```python
from build123d import *

# Parameters (mm, degrees)
F1_DEPTH = 1.5
F2_DEPTH = 0.5
F2_TAPER = 50
F3_DEPTH = 1.5


with BuildPart() as f1:
    # F0 (on Front) → F1 (new body)
    with BuildSketch(Plane.XZ):
        Polygon((-1.5, 1.5), (-20, 1.5), (-22.3259367049, 3), (-28.5, 0), (-22.3259367049, -3), (-20, -1.5), (-1.5, -1.5), (-1.5, -37), (-3, -39.3259400742), (0, -45.5), (3, -39.3259400742), (1.5, -37), (1.5, -1.5), (20, -1.5), (22.3259367049, -3), (28.5, 0), (22.3259367049, 3), (20, 1.5), (1.5, 1.5), (1.5, 23), (3, 25.3259400742), (0, 31.5), (-3, 25.3259400742), (-1.5, 23), align=None)
        Polygon((-1, -1), (-1.5, -1), (-20, -1), (-22.3259367049, -2.5), (-27.4709894508, 0), (-22.3259367049, 2.5), (-20, 1), (-1.5, 1), (-1, 1), (-1, 23), (-2.5, 25.3259400742), (0, 30.4709900124), (2.5, 25.3259400742), (1, 23), (1, 1), (1.5, 1), (20, 1), (22.3259367049, 2.5), (27.4709894508, 0), (22.3259367049, -2.5), (20, -1), (1.5, -1), (1, -1), (1, -37), (2.5, -39.3259400742), (0, -44.4709900124), (-2.5, -39.3259400742), (-1, -37), (-1, -1.5), align=None, mode=Mode.SUBTRACT)
        Polygon((-20, -1), (-1.5, -1), (-1, -1), (-1, -1.5), (-1, -37), (-2.5, -39.3259400742), (0, -44.4709900124), (2.5, -39.3259400742), (1, -37), (1, -1), (1.5, -1), (20, -1), (22.3259367049, -2.5), (27.4709894508, 0), (22.3259367049, 2.5), (20, 1), (1.5, 1), (1, 1), (1, 23), (2.5, 25.3259400742), (0, 30.4709900124), (-2.5, 25.3259400742), (-1, 23), (-1, 1), (-1.5, 1), (-20, 1), (-22.3259367049, 2.5), (-27.4709894508, 0), (-22.3259367049, -2.5), align=None)
    extrude(amount=F1_DEPTH)

    # F0 (on Front) → F2 (join)
    with BuildSketch(Plane.XZ):
        Polygon((-1.5, 1.5), (-20, 1.5), (-22.3259367049, 3), (-28.5, 0), (-22.3259367049, -3), (-20, -1.5), (-1.5, -1.5), (-1.5, -37), (-3, -39.3259400742), (0, -45.5), (3, -39.3259400742), (1.5, -37), (1.5, -1.5), (20, -1.5), (22.3259367049, -3), (28.5, 0), (22.3259367049, 3), (20, 1.5), (1.5, 1.5), (1.5, 23), (3, 25.3259400742), (0, 31.5), (-3, 25.3259400742), (-1.5, 23), align=None)
        Polygon((-1, -1), (-1.5, -1), (-20, -1), (-22.3259367049, -2.5), (-27.4709894508, 0), (-22.3259367049, 2.5), (-20, 1), (-1.5, 1), (-1, 1), (-1, 23), (-2.5, 25.3259400742), (0, 30.4709900124), (2.5, 25.3259400742), (1, 23), (1, 1), (1.5, 1), (20, 1), (22.3259367049, 2.5), (27.4709894508, 0), (22.3259367049, -2.5), (20, -1), (1.5, -1), (1, -1), (1, -37), (2.5, -39.3259400742), (0, -44.4709900124), (-2.5, -39.3259400742), (-1, -37), (-1, -1.5), align=None, mode=Mode.SUBTRACT)
        Polygon((-20, -1), (-1.5, -1), (-1, -1), (-1, -1.5), (-1, -37), (-2.5, -39.3259400742), (0, -44.4709900124), (2.5, -39.3259400742), (1, -37), (1, -1), (1.5, -1), (20, -1), (22.3259367049, -2.5), (27.4709894508, 0), (22.3259367049, 2.5), (20, 1), (1.5, 1), (1, 1), (1, 23), (2.5, 25.3259400742), (0, 30.4709900124), (-2.5, 25.3259400742), (-1, 23), (-1, 1), (-1.5, 1), (-20, 1), (-22.3259367049, 2.5), (-27.4709894508, 0), (-22.3259367049, -2.5), align=None)
    extrude(amount=-F2_DEPTH, taper=F2_TAPER)

    # F3 (add): a face of the model
    f3_faces = [f1.faces().sort_by_distance(p)[0] for p in [
        (0, -1.5, -4.093430874),
    ]]
    extrude(f3_faces, amount=F3_DEPTH)


solid = f1.part
```
Read the model definition and answer for the solid it produces. Units are mm, in the model's axes. A direction names the side the tool comes from. Coordinates: 2 decimals unless noted, no trailing zeros. Write each loop counter-clockwise with the first axis right and the second up, starting at its lowest first coordinate (ties: lowest second). Pieces come first, ordered by that corner, then holes. Notation, with made-up numbers: (-16.75, 21) - (-9.75, 21) arc R30 cw to (-9.75, 53) - close; hole circle Ø1 at (60.25, 20.25). An arc over 180 degrees is marked (long way). Answer as a JSON object with one key per item and string values. Group by question number.
1. Which of the six approach directions +Z, -Z, +X, -X, +Y, -Y give full straight-line access (tool end or side, diameter ignored) to faces 1 (the flat face through (-2.26, -1.48, 24.18)), 2 (the flat face through (2.24, -1.48, 24.15)), 3 (the flat face through (25.456, -1.479, 1.479)), 4 (the flat face through (21.18, -1.48, 2.26))?
2. Consider L1, parallel to X at y = -2.45, z = 2; L2, parallel to X at y = -1.75, z = -36. Determine where each line is inside the solid, lowest interval first. Write a range as [from, to].
3. A cutting plane is placed at A-A (y = -0.75). Determine the outline of the cut face in (x, z).
4. The mould has two halves that part along Z. Classify faces 5 (the flat face through (1.5, -1, -19)), 6 (the flat face through (-1.479, -1.479, 28.456)), 7 (the flat face through (0, -3, -4)), 8 (the flat face through (-25.456, -1.479, -1.479)): +Z half, -Z half, draft (parallel to the pull), parting line (faces both ways), or undercut.
5. Each of these flat-tipped pins is pushed along its axis until it touches: P1, Ø1.5, axis at x = 8.5, y = -2, coming from the -Z side; P2, Ø0.9, axis at y = -2, z = 16, coming from the +X side; P3, Ø1.5, axis at y = -2, z = 9.5, coming from the -X side. Where does it stop, or does it pass through?
Worked out:
{
 "1": {"face 1": "-X, +Y, -Y", "face 2": "+X, +Y, -Y", "face 3": "+Z, +X, +Y, -Y", "face 4": "+Z, +Y, -Y"},
 "2": {"L1": "x = [-24.38, -20.78], [-1.5, 1.5], [20.78, 24.38]", "L2": "x = [-1.5, 1.5]"},
 "3": {"outline": "(-28.5, 0) - (-22.33, -3) - (-20, -1.5) - (-1.5, -1.5) - (-1.5, -37) - (-3, -39.33) - (0, -45.5) - (3, -39.33) - (1.5, -37) - (1.5, -1.5) - (20, -1.5) - (22.33, -3) - (28.5, 0) - (22.33, 3) - (20, 1.5) - (1.5, 1.5) - (1.5, 23) - (3, 25.33) - (0, 31.5) - (-3, 25.33) - (-1.5, 23) - (-1.5, 1.5) - (-20, 1.5) - (-22.33, 3) - close"},
 "4": {"face 5": "undercut", "face 6": "+Z half", "face 7": "draft", "face 8": "-Z half"},
 "5": {"P1": "stops at z = -1.5", "P2": "stops at x = 1.5", "P3": "stops at x = -1.5"}
}
